Autodesk Inventor part; units mm, degrees
ref_plane "YZ Plane" through (0, 0, 0) normal (1, 0, 0) x (0, 1, 0)
ref_plane "XZ Plane" through (0, 0, 0) normal (0, 1, 0) x (-1, 0, 0)
ref_plane "XY Plane" through (0, 0, 0) normal (0, 0, 1) x (1, 0, 0)
sketch "Boceto14" plane through (0, 0, 0) normal (0, 1, 0) x (-1, 0, 0)
  line L0 (39.2545, 8.1893) -> (39.2545, -3.9647)
  line L1 (39.2545, -3.9647) -> (39.2545, 20.0353)
  line L2 (31.2545, 22.0353) -> (-2.7455, 22.0353)
  line L3 (-4.7455, -3.9647) -> (31.2545, -3.9647)
  line L4 (39.2545, 20.0353) -> (39.2545, 30.0353)
  line L5 (39.2545, -3.9647) -> (39.2545, -11.9647)
  circle A0 centre (7.2547, 9.0353) radius 11
  line L6 (-2.7455, 22.0353) -> (-8.7455, 22.0353)
  line L7 (-8.7455, -3.9647) -> (-4.7455, -3.9647)
  line L8 (-8.7455, 22.0353) -> (-10.7455, 22.0353)
  line L9 (-10.7455, 22.0353) -> (-10.7455, -3.9647)
  line L10 (-10.7455, -3.9647) -> (-8.7455, -3.9647)
  circle A1 centre (7.2547, 9.0353) radius 6
  line L11 (39.2545, -11.9647) -> (31.2545, -11.9647)
  line L12 (31.2545, -11.9647) -> (31.2545, -3.9647)
  line L13 (39.2545, 30.0353) -> (31.2545, 30.0353)
  line L14 (31.2545, 30.0353) -> (31.2545, 22.0353)
  point P0 (0, 0)
  dimension "d81" = 42
  dimension "d122" = 22
  dimension "d151" = 2
  dimension "d165" = 31.9998
  dimension "d166" = 12
  dimension "d171" = 13
  dimension "d182" = 8
  dimension "d183" = 8
  dimension "d185" = 8
  dimension "d186" = 8
extrude "Extrusión14" add sketch "Boceto14" along normal blind 40 contours L0 L5 L11 L12 L3 L7 L10 L9 L8 L6 L2 L14 L13 L4 L1 | A0 | A1
sketch "Boceto23" plane through (0, 0, 0) normal (0, -1, 0) x (1, 0, 0)
  point P0 (0, 0)
hole "Agujero1" at (-7.2547, 0, 9.0353) direction (0, 1, 0) diameter 22 depth 40 tip angle 118
extrude "Extrusión20" add sketch "Boceto14" along normal blind 30 contours A0
sketch "Boceto26" plane through (-39.2545, 0, -11.9647) normal (-1, 0, 0) x (0, 0, 1)
  line L0 (42, 0) -> (42, 40)
  line L1 (42, 0) -> (38, 0)
  line L2 (0, 0) -> (42, 0)
  line L3 (38, 0) -> (38, 40)
  line L4 (0, 40) -> (42, 40)
  line L5 (8, 0) -> (0, 0)
  line L6 (0, 0) -> (4, 0)
  line L7 (4, 0) -> (4, 40)
  line L8 (38, 40) -> (38, 30)
  line L9 (38, 30) -> (4, 30)
  line L10 (4, 0) -> (4, 10)
  line L11 (4, 10) -> (38, 10)
  circle A0 centre (38, 10) radius 2
  circle A1 centre (4, 10) radius 2
  circle A2 centre (4, 30) radius 2
  circle A3 centre (38, 30) radius 2
  point P0 (11.9647, 0)
  dimension "d200" = 4
  dimension "d201" = 4
  dimension "d202" = 10
  dimension "d203" = 10
  dimension "d204" = 4
  dimension "d205" = 4
  dimension "d206" = 4
  dimension "d207" = 4
extrude "Extrusión21" cut sketch "Boceto26" against normal blind 30 contours A0 L11 L3 | L3 A0 | A3 L3 | L3 L9 A3 | L11 A0 L3 | L3 A3 L9 | A2 L9 L7 | L7 A2 | A1 L7 | L7 L11 A1 | L11 L7 A1 | A2 L7 L9
thread "Rosca11"
hole "Agujero3" at (-7.2547, 0, 9.0353) direction (0, 1, 0) diameter 14 depth 0.01 tip angle 118
sketch "Boceto27" plane through (0, 40, 0) normal (0, 1, 0) x (1, 0, 0)
  circle A0 centre (-7.2547, -9.0353) radius 6
  line L0 (-7.2547, -9.0353) -> (6.7453, -9.0353)
  line L1 (6.7453, -9.0353) -> (-21.2547, -9.0353)
  circle A1 centre (6.7453, -9.0353) radius 1.5
  circle A2 centre (-21.2547, -9.0353) radius 1.5
  point P0 (0, 0)
  dimension "d226" = 14
  dimension "d227" = 28
  dimension "d228" = 3
  dimension "d229" = 3
hole "Agujero4" at (-21.2547, 40, 9.0353) at (6.7453, 40, 9.0353) direction (0, -1, 0) diameter 3 depth 10 tip angle 118
thread "Rosca12"
thread "Rosca13"
properties part number "Soporte de tuerca de mesa" material "Aluminum 6061"
The listing builds one solid part. Answer for the finished solid, in the listing's coordinates (mm). A direction names the side the tool comes from. Round coordinates to 2 decimals unless told otherwise and drop trailing zeros. Order: outer loops, then holes, each group sorted by start corner. A loop starts at its lowest first (then second) coordinate and runs counter-clockwise, first axis right, second up. Notation, with made-up numbers: (15.5, -5) - (35.5, -5) arc R21 cw to (35.5, 25) - close; hole circle Ø9 at (34.25, 22.25). An arc over 180 degrees is marked (long way). Put each result on its own line as item: value. Start each with the question number.
(1) Find section D-D (y = 17). Give the vertices of the cut face in (x, z), plus the area to 3 significant figures.
(2) Find section A-A (y = 10). Give the vertices of the cut face in (x, z).
(3) Straight lines are drawn through the part: probe 1 along Z at (x, y) = (-35, 30); probe 2 along X at (y, z) = (35, 16); probe 3 along Z at (x, y) = (-17.5, 14). For each, find the intervals that lie inside material, in ascending order. Write a range as from..to.
(4) Determine the mould class of faces 4 (the cylindrical face through (-35.31, 11.35, -9.44)), 5 (the flat face through (-31.254, 20, -8)), 6 (the flat face through (-10, 20, -3.965)) for opening direction Z: released by +Z, released by -Z, zero draft, split by the parting line, or undercut.
(5) For faces 1 (the flat face through (-31.254, 20, 26)), 2 (the flat face through (-39.254, 20, 9)), 3 (the cylindrical face through (-19.79, 34.93, 8.71)), determine the directions among +Z, -Z, +X, -X, +Y, -Y from which every point of the face is accessible in a straight line to the end or side of a thin tool.
(6) Find section B-B (z = 1). Give the vertices of the cut face in (x, y).
(7) Given P1, Ø24, axis at x = -3, z = 5.5, coming from the +Y side; P2, Ø17.5, axis at x = -7.25, z = 9.04, coming from the +Y side; P3, Ø20, axis at x = 0, y = 14.5, coming from the +Z side; P4, Ø10, axis at x = -16.5, y = 32.5, coming from the -Z side, each flat-ended and moving along its own axis, determine where each tip first touches the part or whether it passes through.
(8) Find section C-C (x = 1.5). Give the vertices of the cut face in (y, z), plus the area to 3 significant figures.
Reply:
1. outline: (-39.25, -11.96) - (-31.25, -11.96) - (-31.25, -3.96) - (10.75, -3.96) - (10.75, 22.04) - (-31.25, 22.04) - (-31.25, 30.04) - (-39.25, 30.04) - close; hole circle Ø12 at (-7.25, 9.04)
1. area: 1,310 mm^2
2. outline: (-39.25, -11.96) - (-31.25, -11.96) - (-31.25, -9.96) - (-39.25, -9.96) - close; (-39.25, -5.96) - (-31.25, -5.96) - (-31.25, -3.96) - (10.75, -3.96) - (10.75, 22.04) - (-31.25, 22.04) - (-31.25, 24.04) - (-39.25, 24.04) - close; (-39.25, 28.04) - (-31.25, 28.04) - (-31.25, 30.04) - (-39.25, 30.04) - close; hole circle Ø12 at (-7.25, 9.04)
3. probe 1: -11.96..-9.96, -5.96..24.04, 28.04..30.04
3. probe 2: -39.25..-15.77, 1.26..10.75
3. probe 3: -3.96..22.04
4. face 4: undercut
4. face 5: zero draft
4. face 6: released by -Z
5. face 1: +Z, +X, +Y, -Y
5. face 2: +Z, -Z, -X, +Y, -Y
5. face 3: +Y
6. outline: (-39.25, 0) - (10.75, 0) - (10.75, 40) - (0.26, 40) - (0.26, 30) - (-14.77, 30) - (-14.77, 40) - (-39.25, 40) - close
7. P1: y = 40
7. P2: y = 30
7. P3: z = 22.04
7. P4: z = -3.96
8. outline: (0, -3.96) - (40, -3.96) - (40, 2.38) - (30, 2.38) - (30, 15.7) - (40, 15.7) - (40, 22.04) - (0, 22.04) - close
8. area: 907 mm^2
